The listing builds one solid part. Answer for the finished solid, in the listing's coordinates (mm). A direction names the side the tool comes from. Round coordinates to 2 decimals unless told otherwise and drop trailing zeros. Write each loop counter-clockwise with the first axis right and the second up, starting at its lowest first coordinate (ties: lowest second). Pieces come first, ordered by that corner, then holes. Notation, with made-up numbers: (-35.5, -20.75) - (-31.5, -20.75) arc R29 cw to (-31.5, 4.25) - close; hole circle Ø2 at (74, 39). An arc over 180 degrees is marked (long way). Answer in a Markdown table with one row per item.
from build123d import *

# Parameters (mm, degrees)
SKETCH1_R             = 50
SKETCH1_R_2           = 40
EXTRUDE1_DEPTH        = 60
EXTRUDE2_REACH        = 128.886
EXTRUDE2_END_RADIUS   = 50
EXTRUDE5_DEPTH        = 60
EXTRUDE6_DEPTH        = 149.660687473
EXTRUDE6_DEPTH_BACK   = 149.660687473
SKETCH10_W            = 10
SKETCH10_H            = 4
SKETCH10_H_2          = 0.50125629
EXTRUDE7_DEPTH        = 135.907375632
EXTRUDE8_REACH        = 179.82
SKETCH11_W            = 10
SKETCH11_H            = 15
M8_TAPPED_HOLE2_D     = 6.8
M8_TAPPED_HOLE2_DEPTH = 19.75
M8_TAPPED_HOLE2_TIP   = 2.042926105
M8_TAPPED_HOLE3_D     = 6.8
M8_TAPPED_HOLE3_DEPTH = 19.75
M8_TAPPED_HOLE3_TIP   = 2.042926105


with BuildPart() as part:
    # Sketch1 → Extrude1 (new body)
    with BuildSketch(Plane(origin=(0, 0, 0), x_dir=(1, 0, 0), z_dir=(0, 1, 0))):
        with Locations(Location((0, 0, 0), (0, 0, 270))):
            Circle(SKETCH1_R)
        with Locations(Location((0, 0, 0), (0, 0, 270))):
            Circle(SKETCH1_R_2, mode=Mode.SUBTRACT)
    extrude(amount=EXTRUDE1_DEPTH)

    # Extrude2: up to this cylinder (the profile starts outside it)
    extrude2_end = Plane(origin=(0, 49.27889, 0), z_dir=(0, -1, 0)) * Cylinder(EXTRUDE2_END_RADIUS, 358.772, mode=Mode.PRIVATE)
    # Sketch2 → Extrude2 (add, up to the surface)
    with BuildSketch(Plane.XY.offset(50), mode=Mode.PRIVATE) as extrude2_sk1:
        Polygon((-30, 50), (-20, 50), (-20, 20), (20, 20), (20, 50), (30, 50), (30, 10), (-30, 10), align=None)
    extrude2_tool1 = extrude(extrude2_sk1.sketch, amount=-EXTRUDE2_REACH, mode=Mode.PRIVATE) - extrude2_end
    add(extrude2_tool1.solids().sort_by_distance((-25, 49.27889, 50))[0])
    add(extrude2_tool1.solids().sort_by_distance((-25, 49.27889, 50))[1])

    # Sketch8 → Extrude5 (add)
    with BuildSketch(Plane.XY.offset(50)):
        Polygon((20, 20), (0, 20), (-20, 20), (-20, 50), (-30, 50), (-30, 10), (0, 10), (30, 10), (30, 50), (20, 50), align=None)
    extrude(amount=EXTRUDE5_DEPTH)

    # Sketch9 → Extrude6 (cut, two sides: drawn at the far end of the back side and taken through both)
    with BuildSketch(Plane.ZY.offset(30).offset(-EXTRUDE6_DEPTH_BACK)):
        Polygon((110, 50), (110, 20), (70, 50), align=None)
    extrude(amount=EXTRUDE6_DEPTH + EXTRUDE6_DEPTH_BACK, mode=Mode.SUBTRACT)

    # Sketch10 → Extrude7 (cut, through all)
    with BuildSketch(Plane(origin=(0, 60, 0), x_dir=(1, 0, 0), z_dir=(0, 1, 0))):
        with Locations((0, 40)):
            Rectangle(SKETCH10_W, SKETCH10_H)
        with Locations((0, 50)):
            Rectangle(SKETCH10_W, SKETCH10_H_2)
    extrude(amount=-EXTRUDE7_DEPTH, mode=Mode.SUBTRACT)

    # Sketch11 → Extrude8 (cut, up to next)
    with BuildSketch(Plane(origin=(0, 0, -49.749371855), x_dir=(-1, 0, 0), z_dir=(0, 0, -1)), mode=Mode.PRIVATE) as extrude8_sk1:
        with Locations((0, 30)):
            Rectangle(SKETCH11_W, SKETCH11_H)
    extrude8_tool1 = extrude(extrude8_sk1.sketch, amount=-EXTRUDE8_REACH, mode=Mode.PRIVATE) & part.part
    add(extrude8_tool1.solids().sort_by_distance((0, 30, -49.749372))[0], mode=Mode.SUBTRACT)

    # M8 Tapped Hole2
    with Locations(Plane(origin=(0, 48.75, -49.749371855), x_dir=(-1, 0, 0), z_dir=(0, 0, -1))):
        with Locations((0, 0), (0, -37.5)):
            Hole(M8_TAPPED_HOLE2_D / 2, depth=M8_TAPPED_HOLE2_DEPTH)
            with Locations((0, 0, -(M8_TAPPED_HOLE2_DEPTH + M8_TAPPED_HOLE2_TIP / 2))):  # 118° drill point
                Cone(0, M8_TAPPED_HOLE2_D / 2, M8_TAPPED_HOLE2_TIP, mode=Mode.SUBTRACT)

    # M8 Tapped Hole3
    with Locations(Plane(origin=(-15, 20, 60), x_dir=(0, 0, 1), z_dir=(0, 1, 0))):
        with Locations((0, 0), (0, 30), (40, 0), (40, 30)):
            Hole(M8_TAPPED_HOLE3_D / 2, depth=M8_TAPPED_HOLE3_DEPTH)
            with Locations((0, 0, -(M8_TAPPED_HOLE3_DEPTH + M8_TAPPED_HOLE3_TIP / 2))):  # 118° drill point
                Cone(0, M8_TAPPED_HOLE3_D / 2, M8_TAPPED_HOLE3_TIP, mode=Mode.SUBTRACT)


solid = part.part
(1) Section B-B (x = 25) is taken. Give the vertices of the cut face in (y, z), and give its area (3 significant figures).
Checked values:
| item | result |
|---|---|
| outline | (0, -43.3) - (60, -43.3) - (60, -31.22) - (0, -31.22) - close; (0, 31.22) - (60, 31.22) - (60, 43.3) - (50, 43.3) - (50, 70) - (20, 110) - (10, 110) - (10, 43.3) - (0, 43.3) - close |
| area | 3,520 mm2 |
(2) Section C-C (z = 8.5) is taken. Give the vertices of the cut face in (x, y), and give its area (3 significant figures).
Checked values:
| item | result |
|---|---|
| outline | (-49.27, 0) - (-39.09, 0) - (-39.09, 60) - (-49.27, 60) - close; (39.09, 0) - (49.27, 0) - (49.27, 60) - (39.09, 60) - close |
| area | 1,220 mm2 |
(3) Section D-D (x = 15) is taken. Give the vertices of the cut face in (y, z).
Checked values:
| item | result |
|---|---|
| outline | (0, -47.7) - (60, -47.7) - (60, -37.08) - (0, -37.08) - close; (0, 37.08) - (60, 37.08) - (60, 47.7) - (20, 47.7) - (20, 56.6) - (10, 56.6) - (10, 47.7) - (0, 47.7) - close; (10, 63.4) - (20, 63.4) - (20, 96.6) - (10, 96.6) - close; (10, 103.4) - (20, 103.4) - (20, 110) - (10, 110) - close |
(4) Section A-A (z = 60) is taken. Give the vertices of the cut face in (x, y), and give its area (3 significant figures).
Checked values:
| item | result |
|---|---|
| outline | (-30, 10) - (-18.4, 10) - (-18.4, 20) - (-20, 20) - (-20, 50) - (-30, 50) - close; (-11.6, 10) - (11.6, 10) - (11.6, 20) - (-11.6, 20) - close; (18.4, 10) - (30, 10) - (30, 50) - (20, 50) - (20, 20) - (18.4, 20) - close |
| area | 1,060 mm2 |
(5) Find the intervals of material crossed by line 1 (X direction, y = 17.75, z = 60); line 2 (Y direction, x = 0, z = -44); line 3 (X direction, y = 43.5, z = 56), in increasing order.
Checked values:
| item | result |
|---|---|
| line 1 | x = -30 to -18.4, -11.6 to 11.6, 18.4 to 30 |
| line 2 | y = 0 to 7.85, 14.65 to 22.5, 37.5 to 45.35, 52.15 to 60 |
| line 3 | x = -30 to -20, 20 to 30 |
(6) Flat-ended cylindrical pins translate along their axes: pin 1 (1.5 mm diameter, centred on x = 35.5, y = 9.5, fed in from +Z); pin 2 (3 mm diameter, centred on y = 49, z = 52.5, fed in from +X); pin 3 (3 mm diameter, centred on x = -2, y = 7, fed in from +Z). Find the tip coordinate at first contact, or state that the pin passes through.
Checked values:
| item | result |
|---|---|
| pin 1 | stops at z = 35.95 |
| pin 2 | stops at x = 30 |
| pin 3 | stops at z = 50 |
(7) For a pull along X with two mould halves and no side action, classify faces 1 (the flat face through (-41, 60, -4)), 2 (the flat face through (-3, 14, -42)), 3 (the flat face through (-30, 26, 67)), 4 (the flat face through (-5, 30, -44)) as pulls with the +X half, pulls with the -X half, needs draft (parallel to the pull), parting line crosses it, or undercut.
Checked values:
| item | result |
|---|---|
| face 1 | needs draft |
| face 2 | undercut |
| face 3 | pulls with the -X half |
| face 4 | undercut |
(8) For faces 5 (the flat face through (25, 50, 55)), 6 (the cylindrical face through (-0.44, 52.12, -45.82)), 7 (the cylindrical face through (-16.3, 14.93, 56.86)), 8 (the flat face through (20, 32, 70)), determine the directions among +Z, -Z, +X, -X, +Y, -Y from which every point of the face is accessible in a straight line to the end or side of a thin tool.
Checked values:
| item | result |
|---|---|
| face 5 | +Z, +X, +Y |
| face 6 | -Z |
| face 7 | +Y, -Y |
| face 8 | +Z, +Y |
